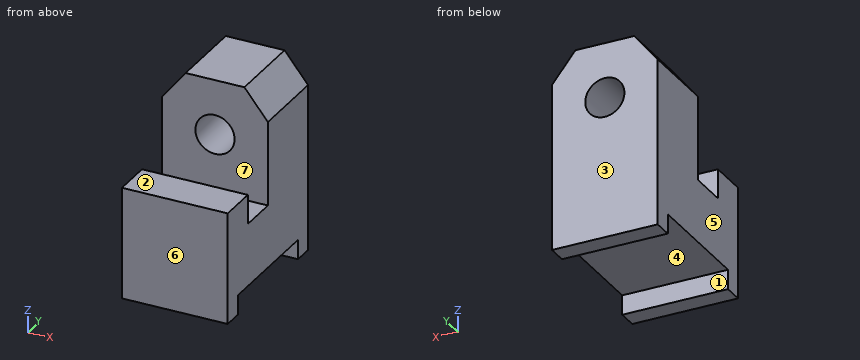
Solid Edge part; units mm, degrees
sketch "Sketch1" plane through (0, 0, 0) normal (1, 0, 0) x (0, 1, 0)
  line L0 (20, 42) -> (20, 57)
  line L1 (20, 57) -> (0, 57)
  line L2 (0, 57) -> (0, 0)
  line L3 (0, 0) -> (10, 0)
  line L4 (10, 0) -> (10, 10)
  line L5 (10, 10) -> (70, 10)
  line L6 (70, 10) -> (70, 0)
  line L7 (70, 0) -> (80, 0)
  line L8 (80, 0) -> (80, 100)
  line L9 (80, 100) -> (40, 100)
  line L10 (40, 100) -> (40, 42)
  line L11 (40, 42) -> (20, 42)
extrude "ExtrudedProtrusion_1" add sketch "Sketch1" against normal blind 54
chamfer "Chamfer_1" distance 12 distance2 15 1 edges at (0, 60, 100) measured on face at (-44.46, 73.7333, 100)
chamfer "Chamfer_2" distance 12 distance2 15 1 edges at (-54, 60, 100) measured on face at (-46.58, 73.7333, 100)
hole "Hole_1" at (-27, 40, 72) direction (0, 1, 0) diameter 20 end up to next
Model file for the job. Use its own axes, mm. Face numbers are marked on the shaded views. A direction names the side the tool comes from. Give positions to 0.01 mm unless a question says otherwise; leave off trailing zeros. Order: outer loops, then holes, each group sorted by start corner. A loop starts at its lowest first (then second) coordinate and runs counter-clockwise, first axis right, second up.
1) Wall check: probe 1 along X at (y, z) = (58, 72); probe 2 along Y at (x, z) = (-14, 55); probe 3 along Z at (x, y) = (-27, 66). Give the ranges that are in metal, low to high.
2) Saw through at D-D, the plane x = -51. Write the cut outline in (y, z), then the cut area to 3 significant figures.
3) Mould opens along Y. For the marked faces 4, 5, 6 and 7 say: +Y half, -Y half, draft (parallel to the pull), parting line (faces both ways), or undercut.
4) Pin check, flat tips, straight feed: pin 1 (23 mm diameter, centred on x = -27, z = 72, fed in from +Y); pin 2 (1 mm diameter, centred on x = -15, y = 37.5, fed in from -Z); pin 3 (10 mm diameter, centred on x = -23.5, y = 32.5, fed in from +Z); pin 4 (16 mm diameter, centred on x = -28.5, y = 9.5, fed in from +Z). Stop position of each tip, or through.
5) Saw through at B-B, the plane y = 45.5. Write the cut outline in (x, z), then the cut area to 3 significant figures.
6) Saw through at C-C, the plane x = -33. Write the cut outline in (y, z).
7) Saw through at A-A, the plane z = 45.5. Write the cut outline in (x, y).
8) 3-axis set-ups, long thin cutter, end or side, ignore diameter. For the marked faces 1, 2 and 3: which of +Z, -Z, +X, -X, +Y, -Y reach the whole face in a straight line?
Computed:
1. probe 1: x = -54 to -37, -17 to 0
1. probe 2: y = 0 to 20, 40 to 80
1. probe 3: z = 10 to 62, 82 to 100
2. outline: (0, 0) - (10, 0) - (10, 10) - (70, 10) - (70, 0) - (80, 0) - (80, 88.75) - (40, 88.75) - (40, 42) - (20, 42) - (20, 57) - (0, 57) - close
2. area: 4,930 mm2
3. face 4: undercut
3. face 5: draft
3. face 6: -Y half
3. face 7: undercut
4. pin 1: stops at y = 80
4. pin 2: stops at z = 10
4. pin 3: stops at z = 42
4. pin 4: stops at z = 57
5. outline: (-54, 10) - (0, 10) - (0, 85) - (-12, 100) - (-42, 100) - (-54, 85) - close; hole circle Ø20 at (-27, 72)
5. area: 4,370 mm2
6. outline: (0, 0) - (10, 0) - (10, 10) - (70, 10) - (70, 0) - (80, 0) - (80, 64) - (40, 64) - (40, 42) - (20, 42) - (20, 57) - (0, 57) - close; (40, 80) - (80, 80) - (80, 100) - (40, 100) - close
7. outline: (-54, 0) - (0, 0) - (0, 20) - (-54, 20) - close; (-54, 40) - (0, 40) - (0, 80) - (-54, 80) - close
8. face 1: -Z, +X, -X
8. face 2: +Z, +X, -X, -Y
8. face 3: +Z, -Z, +X, -X, +Y
